```python
from build123d import *

# Parameters (mm, degrees)
F1_DEPTH = 3


with BuildPart() as f1:
    # F0 (on Top) → F1 (new body)
    with BuildSketch(Plane.XY):
        with BuildLine():
            ThreePointArc((37.418773, -2.466863), (37.479688, -1.2341), (37.5, 0))
            ThreePointArc((37.5, 0), (37.479688, 1.2341), (37.418773, 2.466863))
            ThreePointArc((37.418773, 2.466863), (37.038313, 5.866292), (36.349671, 9.21691))
            ThreePointArc((36.349671, 9.21691), (35.664619, 11.588137), (34.825065, 13.909163))
            ThreePointArc((34.825065, 13.909163), (33.412745, 17.024644), (31.722409, 19.998469))
            ThreePointArc((31.722409, 19.998469), (30.338137, 22.041947), (28.822438, 23.989937))
            ThreePointArc((28.822438, 23.989937), (26.516504, 26.516504), (23.989937, 28.822438))
            ThreePointArc((23.989937, 28.822438), (22.041947, 30.338137), (19.998469, 31.722409))
            ThreePointArc((19.998469, 31.722409), (17.024644, 33.412745), (13.909163, 34.825065))
            ThreePointArc((13.909163, 34.825065), (11.588137, 35.664619), (9.21691, 36.349671))
            ThreePointArc((9.21691, 36.349671), (5.866292, 37.038313), (2.466863, 37.418773))
            ThreePointArc((2.466863, 37.418773), (0, 37.5), (-2.466863, 37.418773))
            ThreePointArc((-2.466863, 37.418773), (-5.866292, 37.038313), (-9.21691, 36.349671))
            ThreePointArc((-9.21691, 36.349671), (-11.588137, 35.664619), (-13.909163, 34.825065))
            ThreePointArc((-13.909163, 34.825065), (-17.024644, 33.412745), (-19.998469, 31.722409))
            ThreePointArc((-19.998469, 31.722409), (-22.041947, 30.338137), (-23.989937, 28.822438))
            ThreePointArc((-23.989937, 28.822438), (-26.516504, 26.516504), (-28.822438, 23.989937))
            ThreePointArc((-28.822438, 23.989937), (-30.338137, 22.041947), (-31.722409, 19.998469))
            ThreePointArc((-31.722409, 19.998469), (-33.412745, 17.024644), (-34.825065, 13.909163))
            ThreePointArc((-34.825065, 13.909163), (-35.664619, 11.588137), (-36.349671, 9.21691))
            ThreePointArc((-36.349671, 9.21691), (-37.038313, 5.866292), (-37.418773, 2.466863))
            ThreePointArc((-37.418773, 2.466863), (-37.5, 0), (-37.418773, -2.466863))
            ThreePointArc((-37.418773, -2.466863), (-37.038313, -5.866292), (-36.349671, -9.21691))
            ThreePointArc((-36.349671, -9.21691), (-35.664619, -11.588137), (-34.825065, -13.909163))
            ThreePointArc((-34.825065, -13.909163), (-33.412745, -17.024644), (-31.722409, -19.998469))
            ThreePointArc((-31.722409, -19.998469), (-30.338137, -22.041947), (-28.822438, -23.989937))
            ThreePointArc((-28.822438, -23.989937), (-26.516504, -26.516504), (-23.989937, -28.822438))
            ThreePointArc((-23.989937, -28.822438), (-22.041947, -30.338137), (-19.998469, -31.722409))
            ThreePointArc((-19.998469, -31.722409), (-17.024644, -33.412745), (-13.909163, -34.825065))
            ThreePointArc((-13.909163, -34.825065), (-11.588137, -35.664619), (-9.21691, -36.349671))
            ThreePointArc((-9.21691, -36.349671), (-5.866292, -37.038313), (-2.466863, -37.418773))
            ThreePointArc((-2.466863, -37.418773), (0, -37.5), (2.466863, -37.418773))
            ThreePointArc((2.466863, -37.418773), (5.866292, -37.038313), (9.21691, -36.349671))
            ThreePointArc((9.21691, -36.349671), (11.588137, -35.664619), (13.909163, -34.825065))
            ThreePointArc((13.909163, -34.825065), (17.024644, -33.412745), (19.998469, -31.722409))
            ThreePointArc((19.998469, -31.722409), (22.041947, -30.338137), (23.989937, -28.822438))
            ThreePointArc((23.989937, -28.822438), (26.516504, -26.516504), (28.822438, -23.989937))
            ThreePointArc((28.822438, -23.989937), (30.338137, -22.041947), (31.722409, -19.998469))
            ThreePointArc((31.722409, -19.998469), (33.412745, -17.024644), (34.825065, -13.909163))
            ThreePointArc((34.825065, -13.909163), (35.664619, -11.588137), (36.349671, -9.21691))
            ThreePointArc((36.349671, -9.21691), (37.038313, -5.866292), (37.418773, -2.466863))
        make_face()
        with BuildLine():
            ThreePointArc((37.418773, 2.466863), (37.479688, 1.2341), (37.5, 0))
            ThreePointArc((37.5, 0), (37.479688, -1.2341), (37.418773, -2.466863))
            Line((37.418773, -2.466863), (41.188397, 0))
            Line((41.188397, 0), (37.418773, 2.466863))
        make_face()
        with BuildLine():
            ThreePointArc((34.825065, 13.909163), (35.664619, 11.588137), (36.349671, 9.21691))
            Line((36.349671, 9.21691), (39.172493, 12.727915))
            Line((39.172493, 12.727915), (34.825065, 13.909163))
        make_face()
        with BuildLine():
            Line((39.172493, -12.727915), (36.349671, -9.21691))
            ThreePointArc((36.349671, -9.21691), (35.664619, -11.588137), (34.825065, -13.909163))
            Line((34.825065, -13.909163), (39.172493, -12.727915))
        make_face()
        with BuildLine():
            ThreePointArc((28.822438, 23.989937), (30.338137, 22.041947), (31.722409, 19.998469))
            Line((31.722409, 19.998469), (33.322113, 24.209932))
            Line((33.322113, 24.209932), (28.822438, 23.989937))
        make_face()
        with BuildLine():
            Line((33.322113, -24.209932), (31.722409, -19.998469))
            ThreePointArc((31.722409, -19.998469), (30.338137, -22.041947), (28.822438, -23.989937))
            Line((28.822438, -23.989937), (33.322113, -24.209932))
        make_face()
        with BuildLine():
            ThreePointArc((19.998469, 31.722409), (22.041947, 30.338137), (23.989937, 28.822438))
            Line((23.989937, 28.822438), (24.209932, 33.322113))
            Line((24.209932, 33.322113), (19.998469, 31.722409))
        make_face()
        with BuildLine():
            Line((24.209932, -33.322113), (23.989937, -28.822438))
            ThreePointArc((23.989937, -28.822438), (22.041947, -30.338137), (19.998469, -31.722409))
            Line((19.998469, -31.722409), (24.209932, -33.322113))
        make_face()
        with BuildLine():
            ThreePointArc((9.21691, 36.349671), (11.588137, 35.664619), (13.909163, 34.825065))
            Line((13.909163, 34.825065), (12.727915, 39.172493))
            Line((12.727915, 39.172493), (9.21691, 36.349671))
        make_face()
        with BuildLine():
            Line((12.727915, -39.172493), (13.909163, -34.825065))
            ThreePointArc((13.909163, -34.825065), (11.588137, -35.664619), (9.21691, -36.349671))
            Line((9.21691, -36.349671), (12.727915, -39.172493))
        make_face()
        with BuildLine():
            ThreePointArc((-2.466863, 37.418773), (0, 37.5), (2.466863, 37.418773))
            Line((2.466863, 37.418773), (0, 41.188397))
            Line((0, 41.188397), (-2.466863, 37.418773))
        make_face()
        with BuildLine():
            Line((0, -41.188397), (2.466863, -37.418773))
            ThreePointArc((2.466863, -37.418773), (0, -37.5), (-2.466863, -37.418773))
            Line((-2.466863, -37.418773), (0, -41.188397))
        make_face()
        with BuildLine():
            ThreePointArc((-13.909163, 34.825065), (-11.588137, 35.664619), (-9.21691, 36.349671))
            Line((-9.21691, 36.349671), (-12.727915, 39.172493))
            Line((-12.727915, 39.172493), (-13.909163, 34.825065))
        make_face()
        with BuildLine():
            Line((-12.727915, -39.172493), (-9.21691, -36.349671))
            ThreePointArc((-9.21691, -36.349671), (-11.588137, -35.664619), (-13.909163, -34.825065))
            Line((-13.909163, -34.825065), (-12.727915, -39.172493))
        make_face()
        with BuildLine():
            ThreePointArc((-23.989937, 28.822438), (-22.041947, 30.338137), (-19.998469, 31.722409))
            Line((-19.998469, 31.722409), (-24.209932, 33.322113))
            Line((-24.209932, 33.322113), (-23.989937, 28.822438))
        make_face()
        with BuildLine():
            Line((-24.209932, -33.322113), (-19.998469, -31.722409))
            ThreePointArc((-19.998469, -31.722409), (-22.041947, -30.338137), (-23.989937, -28.822438))
            Line((-23.989937, -28.822438), (-24.209932, -33.322113))
        make_face()
        with BuildLine():
            ThreePointArc((-31.722409, 19.998469), (-30.338137, 22.041947), (-28.822438, 23.989937))
            Line((-28.822438, 23.989937), (-33.322113, 24.209932))
            Line((-33.322113, 24.209932), (-31.722409, 19.998469))
        make_face()
        with BuildLine():
            Line((-33.322113, -24.209932), (-28.822438, -23.989937))
            ThreePointArc((-28.822438, -23.989937), (-30.338137, -22.041947), (-31.722409, -19.998469))
            Line((-31.722409, -19.998469), (-33.322113, -24.209932))
        make_face()
        with BuildLine():
            ThreePointArc((-36.349671, 9.21691), (-35.664619, 11.588137), (-34.825065, 13.909163))
            Line((-34.825065, 13.909163), (-39.172493, 12.727915))
            Line((-39.172493, 12.727915), (-36.349671, 9.21691))
        make_face()
        with BuildLine():
            Line((-39.172493, -12.727915), (-34.825065, -13.909163))
            ThreePointArc((-34.825065, -13.909163), (-35.664619, -11.588137), (-36.349671, -9.21691))
            Line((-36.349671, -9.21691), (-39.172493, -12.727915))
        make_face()
        with BuildLine():
            ThreePointArc((-37.418773, -2.466863), (-37.5, 0), (-37.418773, 2.466863))
            Line((-37.418773, 2.466863), (-41.188397, 0))
            Line((-41.188397, 0), (-37.418773, -2.466863))
        make_face()
    extrude(amount=F1_DEPTH)


solid = f1.part
```
Geometry check sheet. Reference: the model listing, model coordinates, mm. A direction names the side the tool comes from. Give positions to 0.01 mm unless a question says otherwise; leave off trailing zeros. Loops run counter-clockwise (first coordinate to the right, second up) from the corner with the lowest first, then second, coordinate; pieces in that order, holes last. Notation, with made-up numbers: M 83.25,-11 L 123.25,-11 A5 cw 123.25,-5 Z; hole C 77.5,-37 d6. An arc over 180 degrees is marked long. Write item = value, one per line.
(1) Sectioned sample at A-A, the plane x = -18.5. Record the cut outline in (y, z), plus the area to 3 significant figures.
Answer below:
outline = M -32.62,0 L 32.62,0 L 32.62,3 L -32.62,3 Z
area = 196 mm2
(2) Gauge pin test, flat ends, axial feed: pin 1 Ø1 at (y, z) = (20.5, 2.5) entering from +X; pin 2 Ø1.5 at (y, z) = (-27, 2.5) entering from +X; pin 3 Ø1.5 at (y, z) = (-16, 0.5) entering from -X. Record the tip position at first contact, or that the pin passes through.
Answer below:
pin_1 = 32.1
pin_2 = 26.78
pin_3 = -34.26
(3) Release check for a two-part mould opening along Y. For faces 1 (the face through (10.997, 37.781, 1.479)), 2 (the face through (-31.1, -24.1, 1.5)), 3 (the face through (-39.33, -1.216, 1.479)), 4 (the face through (-1, 1, 0)) record: released by +Y, released by -Y, zero draft, split by the parting line, or undercut.
Answer below:
face_1 = released by +Y
face_2 = released by -Y
face_3 = undercut
face_4 = zero draft
(4) Tool access check on faces 5 (the face through (22.07, -32.51, 1.48)), 6 (the face through (22.13, 32.53, 1.48)), 7 (the face through (37.03, -5.91, 1.48)), 8 (the face through (-37.046, -5.819, 1.479)). Record the directions out of +Z, -Z, +X, -X, +Y, -Y that give a thin tool (end or side, any length) a straight path to the whole face; none if there is none.
Answer below:
face_5 = +Z, -Z, -Y
face_6 = +Z, -Z, +Y
face_7 = +Z, -Z, +X
face_8 = +Z, -Z, -X
(5) Material ranges on line 1 (Y direction, x = -2.5, z = 2.3); line 2 (X direction, y = 12, z = 1.95); line 3 (Y direction, x = 28.5, z = 1.15), recorded low to high. Write a range as [from, to].
Answer below:
line_1 = [-37.42, 37.42]
line_2 = [-38.59, 38.59]
line_3 = [-24.37, 24.37]
(6) Sectioned sample at B-B, the plane y = 16.5. Record the cut outline in (x, z), plus the area to 3 significant figures.
Answer below:
outline = M -33.67,0 L 33.67,0 L 33.67,3 L -33.67,3 Z
area = 202 mm2
